Build history of the part. All positions in model axes, mm. Round coordinates to 2 decimals unless told otherwise and drop trailing zeros. Write each loop counter-clockwise with the first axis right and the second up, starting at its lowest first coordinate (ties: lowest second). Pieces come first, ordered by that corner, then holes. Notation, with made-up numbers: (58.25, 9.25) -> (91.25, 9.25) arc R27 cw to (91.25, 32.25) -> close; hole circle Ø10 at (-5.5, 87.25). An arc over 180 degrees is marked (long way). Return JSON: item names as keys, results as strings.
Autodesk Inventor part; units mm, degrees
ref_plane "YZ Plane" through (0, 0, 0) normal (1, 0, 0) x (0, 1, 0)
ref_plane "XZ Plane" through (0, 0, 0) normal (0, 1, 0) x (-1, 0, 0)
ref_plane "XY Plane" through (0, 0, 0) normal (0, 0, 1) x (1, 0, 0)
sketch "Sketch1" plane through (0, 0, 0) normal (0, 0, 1) x (1, 0, 0)
  line L0 (0, 0) -> (14, 0)
  line L1 (14, 0) -> (14, 35)
  line L2 (14, 35) -> (0, 35)
  line L3 (0, 35) -> (0, 0)
  dimension "d0" = 14
  dimension "d1" = 35
extrude "Extrusion1" add sketch "Sketch1" along normal blind 3
sketch "Sketch2" plane through (0, 0, 3) normal (0, 0, 1) x (1, 0, 0)
  line L0 (0, 0) -> (0, 35)
  line L1 (0, 35) -> (14, 35)
  point P0 (7, 22)
  dimension "d4" = 13
  dimension "d5" = 7
hole "Hole1" at (7, 22, 3) direction (0, 0, -1) diameter 6.5 depth 3 tip angle 118 countersink diameter 11.5 countersink angle 90
sketch "Sketch3" plane through (0, 0, 0) normal (0, 0, -1) x (-1, 0, 0)
  line L0 (0, 0) -> (-14, 0)
  line L1 (0, 35) -> (0, 0)
  point P0 (-7, 7)
  dimension "d13" = 7
  dimension "d14" = 7
hole "Hole2" at (7, 7, 0) direction (0, 0, 1) diameter 3.2 depth 3 tip angle 118 countersink diameter 4 countersink angle 90
properties part number "SUPORTE(44)" material "Carbon Steel"
Q1. Wall check: L1, parallel to Y at x = 7, z = 0.45; L2, parallel to X at y = 7, z = 1.15; L3, parallel to X at y = 22, z = 0.4. Give the ranges that are in metal, low to high.
Verdict:
{"L1": "y = 0 to 5.4, 8.6 to 18.75, 25.25 to 35", "L2": "x = 0 to 5.4, 8.6 to 14", "L3": "x = 0 to 3.75, 10.25 to 14"}
Q2. Saw through at C-C on z = 1.75. List the corners of the cut face in (x, y), then the cut area to 3 significant figures.
Verdict:
{"outline": "(0, 0) -> (14, 0) -> (14, 35) -> (0, 35) -> close; hole circle Ø9 at (7, 22); hole circle Ø3.2 at (7, 7)", "area": "418 mm²"}
Q3. Saw through at B-B on y = 22. List the corners of the cut face in (x, z), then the cut area to 4 significant figures.
Verdict:
{"outline": "(0, 0) -> (3.75, 0) -> (3.75, 0.5) -> (1.25, 3) -> (0, 3) -> close; (10.25, 0) -> (14, 0) -> (14, 3) -> (12.75, 3) -> (10.25, 0.5) -> close", "area": "16.25 mm²"}
Q4. Saw through at D-D on y = 7. List the corners of the cut face in (x, z), then the cut area to 3 significant figures.
Verdict:
{"outline": "(0, 0) -> (5, 0) -> (5.4, 0.4) -> (5.4, 3) -> (0, 3) -> close; (8.6, 0.4) -> (9, 0) -> (14, 0) -> (14, 3) -> (8.6, 3) -> close", "area": "32.2 mm²"}
Q5. Pin check, flat tips, straight feed: pin 1 Ø7.5 at (x, y) = (7, 22) entering from +Z; pin 2 Ø1.9 at (x, y) = (7, 7) entering from +Z. Stop position of each tip, or through.
Verdict:
{"pin 1": "stops at z = 1", "pin 2": "passes through"}
Q6. Two-plate mould, pull along Y, no slides. Class faces 1 (the flat face through (14, 17, 1)), 2 (the cylindrical face through (8.56, 6.65, 1.72)), 3 (the flat face through (7, 0, 1)): +Y half, -Y half, draft (parallel to the pull), parting line (faces both ways), or undercut.
Verdict:
{"face 1": "draft", "face 2": "undercut", "face 3": "-Y half"}
Q7. Saw through at A-A on x = 7. List the corners of the cut face in (y, z).
Verdict:
{"outline": "(0, 0) -> (5, 0) -> (5.4, 0.4) -> (5.4, 3) -> (0, 3) -> close; (8.6, 0.4) -> (9, 0) -> (18.75, 0) -> (18.75, 0.5) -> (16.25, 3) -> (8.6, 3) -> close; (25.25, 0) -> (35, 0) -> (35, 3) -> (27.75, 3) -> (25.25, 0.5) -> close"}
